Study the drawing (mm; zero at the part's minimum x, y, z) and answer. A direction names the side the tool comes from. Coordinates: 2 decimals unless noted, no trailing zeros. Write each loop counter-clockwise with the first axis right and the second up, starting at its lowest first coordinate (ties: lowest second). Pieces come first, ordered by that corner, then holes. Notation, with made-up numbers: M -3,-22.75 L 23,-22.75 A26 ccw 23,-3.75 Z; hole C 49.25,12 d11. An arc over 180 degrees is marked long. Answer as CSV lines item,"result". Start each with the question number.
(1) Find the intervals of material crossed by L1, parallel to X at y = 3.25, z = 12; L2, parallel to Y at x = 3, z = 6.25; L3, parallel to Z at x = 12.25, y = 14 (1 decimal), in increasing order. Write a range as [from, to].
(2) A cutting plane is placed at D-D on x = 7.5. Give the vertices of the cut face in (y, z) (1 decimal), then the cut area to 3 significant figures.
(3) Flat-ended cylindrical pins translate along their axes: P1, Ø2, axis at x = 20.5, z = 4.5, coming from the -Y side; P2, Ø2, axis at y = 14, z = 15.5, coming from the -X side; P3, Ø2, axis at y = 17.5, z = 7, coming from the +X side (1 decimal). Find the tip coordinate at first contact, or state that the pin passes through.
(4) A cutting plane is placed at B-B on z = 12. Give the vertices of the cut face in (x, y).
(5) For the marked faces 1, 2 and 3, determine the directions among +Z, -Z, +X, -X, +Y, -Y from which every point of the face is accessible in a straight line to the end or side of a thin tool.
(6) A cutting plane is placed at C-C on y = 21. Give the vertices of the cut face in (x, z), then the cut area to 3 significant figures.
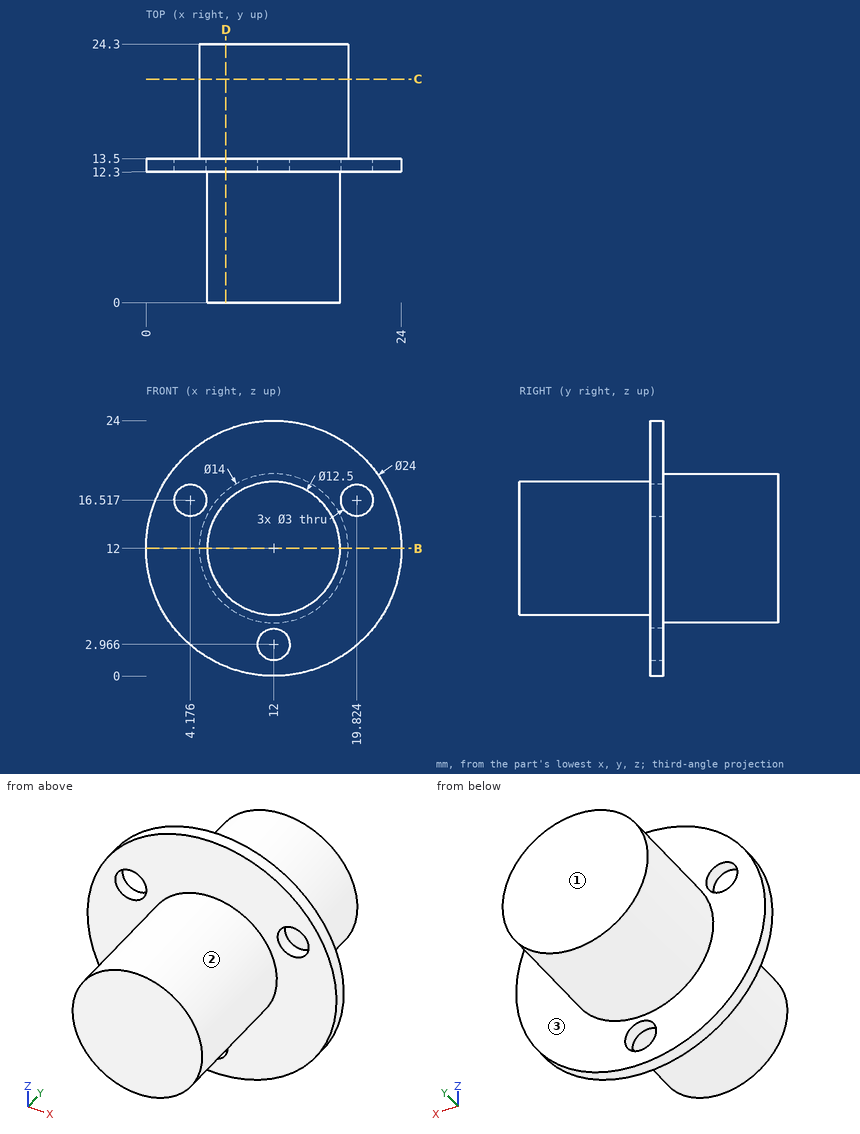
Here are the results:
1,L1,"x = [5.75, 18.25]"
1,L2,"y = [12.3, 13.5]"
1,L3,"z = [5, 19]"
2,outline,"M 0,7.7 L 12.3,7.7 L 12.3,0.9 L 13.5,0.9 L 13.5,6.6 L 24.3,6.6 L 24.3,17.4 L 13.5,17.4 L 13.5,23.1 L 12.3,23.1 L 12.3,16.3 L 0,16.3 Z"
2,area,"249 mm^2"
3,P1,"stops at y = 12.3"
3,P2,"stops at x = 0.29"
3,P3,"stops at x = 17.7"
4,outline,"M 0,12.3 L 5.75,12.3 L 5.75,0 L 18.25,0 L 18.25,12.3 L 24,12.3 L 24,13.5 L 19,13.5 L 19,24.3 L 5,24.3 L 5,13.5 L 0,13.5 Z"
5,face 1,"+Z, -Z, +X, -X, +Y"
5,face 2,"-Y"
5,face 3,"+Y"
6,outline,"C 12,12 d14"
6,area,"154 mm^2"
